```python
from build123d import *

# Parameters (mm, degrees)
F1_DEPTH = 3


with BuildPart() as f1:
    # F0 (on Front) → F1 (new body)
    with BuildSketch(Plane.XZ):
        Polygon((100.7, -25), (121, -25), (121, -10), (118, -10), (118, 10), (121, 10), (121, 25), (100.7, 25), (100.7, 28), (100.7, 31), (60.7, 31), (60.7, 28), (60.7, 25), (20, 25), (20, 28), (20, 31), (-20, 31), (-20, 28), (-20, 25), (-60.7, 25), (-60.7, 28), (-60.7, 31), (-100.7, 31), (-100.7, 28), (-100.7, 25), (-121, 25), (-121, 10), (-118, 10), (-118, -10), (-121, -10), (-121, -25), (-100.7, -25), (-100.7, -28), (-60.7, -28), (-60.7, -25), (-20, -25), (-20, -28), (20, -28), (20, -25), (60.7, -25), (60.7, -28), (100.7, -28), align=None)
    extrude(amount=F1_DEPTH)


solid = f1.part
```
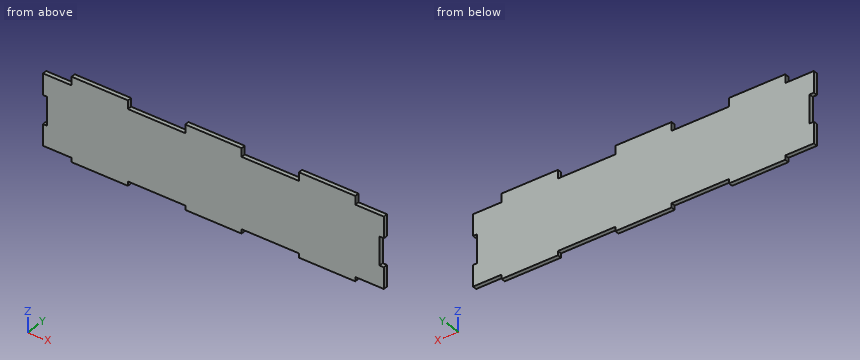
Geometry: final body of the model. Coordinates: model frame, mm. Coordinates: 2 decimals unless noted, no trailing zeros. Order: outer loops, then holes, each group sorted by start corner. A loop starts at its lowest first (then second) coordinate and runs counter-clockwise, first axis right, second up.
Item 1: Material intervals for line 1 along X through (y, z) = (-1.35, 29.5); line 2 along Z through (x, y) = (-46, -0.35); line 3 along X through (y, z) = (-0.45, 7), sorted ascending.
Answer:
line 1: x = -100.7 to -60.7, -20 to 20, 60.7 to 100.7
line 2: z = -25 to 25
line 3: x = -118 to 118
Item 2: Section query B-B (x = -58). Output: boundary loops of the cut face in (y, z).
Answer:
outline: (-3, -25) - (0, -25) - (0, 25) - (-3, 25) - close
Item 3: Contact query for flat-ended pins moving along their axis: P1, Ø1.5, axis at x = 50, y = -1, coming from the -Z side; P2, Ø1.5, axis at y = -1.5, z = -27, coming from the +X side; P3, Ø0.9, axis at x = 42, y = -1, coming from the +Z side; P4, Ø6, axis at x = -19.5, z = -5, coming from the +Y side. Output: stop coordinate, or through.
Answer:
P1: stops at z = -25
P2: stops at x = 100.7
P3: stops at z = 25
P4: stops at y = 0
Item 4: Section query A-A (z = -2). Output: boundary loops of the cut face in (x, y).
Answer:
outline: (-118, -3) - (118, -3) - (118, 0) - (-118, 0) - close
